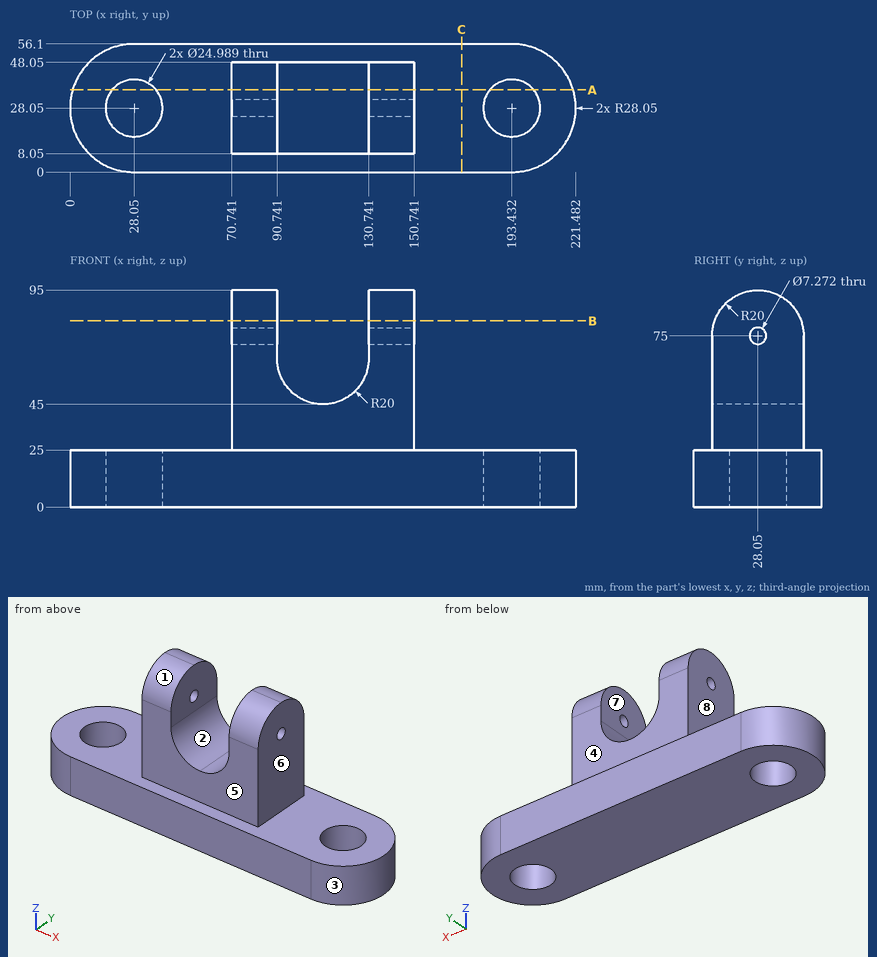
Study the drawing (mm; zero at the part's minimum x, y, z) and answer. A direction names the side the tool comes from. Round coordinates to 2 decimals unless told otherwise and drop trailing zeros. Loops run counter-clockwise (first coordinate to the right, second up) from the corner with the lowest first, then second, coordinate; pieces in that order, holes last. Notation, with made-up numbers: (52, -1.5) -> (76, -1.5) arc R8 cw to (76, 6.5) -> close; hole circle Ø3 at (86.5, 84). An arc over 180 degrees is marked (long way). Use one line per item in the form item = value.
1. The part is cut by section A-A on y = 36. Give the number of separate pieces and of enclosed holes in the cut face, and give its area (3 significant figures).
Answer key:
separate_pieces = 3
enclosed_holes = 0
area = 8,220 mm²
2. A tool of negligible diameter and unlimited length cuts with its end or side. For the marked faces 4, 5, 6, 7 and 8, from which of +Z, -Z, +X, -X, +Y, -Y can it reach the whole face along a straight path? Write none if from no direction.
Answer key:
face_4 = +Z, +X, -X, +Y
face_5 = +Z, +X, -X, -Y
face_6 = +Z, +X, +Y, -Y
face_7 = +Z, +Y, -Y
face_8 = +Z, -X, +Y, -Y
3. The part is cut by section C-C on x = 171.5. Determine the outline of the cut face in (y, z), and give its area (3 significant figures).
Answer key:
outline = (0, 0) -> (56.1, 0) -> (56.1, 25) -> (0, 25) -> close
area = 1,400 mm²
4. Flat-ended cylindrical pins translate along their axes: pin 1 Ø9 at (y, z) = (22, 83.5) entering from -X; pin 2 Ø4 at (x, z) = (196.5, 10) entering from +Y; pin 3 Ø15 at (x, z) = (126.5, 42) entering from -Y. Find the tip coordinate at first contact, or state that the pin passes through.
Answer key:
pin_1 = 70.74
pin_2 = 56.08
pin_3 = 8.05
5. The part is cut by section B-B on z = 81.5. Determine the outline of the cut face in (x, y).
Answer key:
outline = (70.74, 9.14) -> (90.74, 9.14) -> (90.74, 46.96) -> (70.74, 46.96) -> close; (130.74, 9.14) -> (150.74, 9.14) -> (150.74, 46.96) -> (130.74, 46.96) -> close
6. For a pull along X with two mould halves and no side action, classify the marked faces 1, 2 and 3 as released by +X, released by -X, zero draft, split by the parting line, or undercut.
Answer key:
face_1 = zero draft
face_2 = undercut
face_3 = released by +X
7. Find the intervals of material crossed by probe 1 along X at (y, z) = (45.5, 82); probe 2 along Y at (x, z) = (77.5, 75.5); probe 3 along Z at (x, y) = (193, 11), in increasing order. Write a range as [from, to].
Answer key:
probe_1 = [70.74, 90.74], [130.74, 150.74]
probe_2 = [8.06, 24.45], [31.65, 48.04]
probe_3 = [0, 25]
